For this review, take the finished solid that the model builds, in its own axes (mm). A direction names the side the tool comes from. Coordinates: 2 decimals unless noted, no trailing zeros. Order: outer loops, then holes, each group sorted by start corner. A loop starts at its lowest first (then second) coordinate and runs counter-clockwise, first axis right, second up. Notation, with made-up numbers: (79.5, 36.25) -> (109.5, 36.25) arc R11 cw to (109.5, 44.25) -> close; hole circle Ø11 at (18.5, 41). An arc over 180 degrees is marked (long way). Return JSON: item names as keys, results as strings. Group by question number.
Item 1: Take a section at B-B (x = -55). Write out the cut boundary in (y, z).
Item 2: Take a section at C-C (z = -149). Write out the cut boundary in (x, y), then the cut area to 3 significant figures.
Item 3: Take a section at D-D (z = -42). Write out the cut boundary in (x, y), then the cut area to 3 significant figures.
Item 4: Insertion check: pin 1 (5 mm diameter, centred on x = 42.5, z = -57.5, fed in from +Y); pin 2 (10 mm diameter, centred on x = -15.5, y = -2, fed in from -Z); pin 3 (11 mm diameter, centred on y = 0, z = -42, fed in from -X); pin 4 (12 mm diameter, centred on y = 2, z = -137.5, fed in from +X). Each pin has a flat end and moves straight along its axis. Give the tip position at first contact, or say it passes through.
Item 5: Take a section at A-A (z = -126). Write out the cut boundary in (x, y).
Item 6: Machinability: for faces 4 (the cylindrical face through (39.96, -1.76, -161.75)), 5 (the cylindrical face through (-94, 0, -120)), 6 (the flat face through (-28, 28, -12)), which of the approach directions +Z, -Z, +X, -X, +Y, -Y give a long, thin tool a straight path to every point of the face, cutting with its end or side? Answer none if there is none.
Item 7: For line 1 along Y through (x, z) = (0, -169.5); line 2 along Z through (x, y) = (-28, -46.5); line 3 along Y through (x, z) = (11.5, -62), list the stretches that pass through material, from the lowest coordinate up.
Item 8: Draft analysis for pull direction Y (two halves, no side actions). For faces 1 (the cylindrical face through (-60, 0, -6)), 2 (the flat face through (32, 42, -166)), 3 (the cylindrical face through (-62.952, -19.825, -6.084)), state which applies: +Y half, -Y half, draft (parallel to the pull), parting line (faces both ways), or undercut.
```python
from build123d import *
from build123d.topology import SkipClean

# Parameters (mm, degrees)
SKETCH4_R          = 6
CUT_EXTRUDE1_DEPTH = 12
SKETCH5_R          = 6
CUT_EXTRUDE2_DEPTH = 14
SKETCH14_R         = 6
CUT_EXTRUDE3_DEPTH = 12


with BuildPart() as part:
    # Sketch1 → Revolve1 (revolve)
    with BuildSketch(Plane(origin=(0, 0, 0), x_dir=(1, 0, 0), z_dir=(0, 1, 0)), mode=Mode.PRIVATE) as revolve1_sk:
        Polygon((40, 180), (40, 144), (27, 36), (20, 36), (20, 0), (66, 0), (66, 12), (36, 12), (36, 36), (50, 144), (52, 144), (52, 166), (72, 166), (72, 180), align=None)
    revolve(revolve1_sk.sketch.rotate(Axis((0, 0, -182.979971196), (0, 0, 1)), 180), axis=Axis((0, 0, -182.979971196), (0, 0, 1)))

    # Sketch4 → Cut-Extrude1 (cut)
    with BuildSketch(Plane.XY):
        with Locations((54, 0)):
            Circle(SKETCH4_R)
        with Locations((0, -54)):
            Circle(SKETCH4_R)
        with Locations((-54, 0)):
            Circle(SKETCH4_R)
        with Locations((0, 54)):
            Circle(SKETCH4_R)
    extrude(amount=-CUT_EXTRUDE1_DEPTH, mode=Mode.SUBTRACT)

    # Sketch5 → Cut-Extrude2 (cut)
    with BuildSketch(Plane(origin=(0, 0, -180), x_dir=(-1, 0, 0), z_dir=(0, 0, -1))):
        with Locations((58, 0)):
            Circle(SKETCH5_R)
        with Locations((0, -58)):
            Circle(SKETCH5_R)
        with Locations((-58, 0)):
            Circle(SKETCH5_R)
        with Locations((0, 58)):
            Circle(SKETCH5_R)
    extrude(amount=-CUT_EXTRUDE2_DEPTH, mode=Mode.SUBTRACT)

    # Sketch11 → Revolve2 (revolve)
    with BuildSketch(Plane(origin=(0, 0, 0), x_dir=(1, 0, 0), z_dir=(0, 1, 0)), mode=Mode.PRIVATE) as revolve2_sk:
        Polygon((0, 54.187764991), (-100, 64), (-100, 28), (-88, 28), (-88, 52.774507139), (0, 44.139740331), align=None)
    revolve(revolve2_sk.sketch.rotate(Axis((-156.93032519, 0, -84), (1, 0, 0)), 142.376659073), axis=Axis((-156.93032519, 0, -84), (1, 0, 0)))

    # Sketch12 → Cut-Revolve1 (revolve, cut)
    with BuildSketch(Plane(origin=(0, 0, 0), x_dir=(1, 0, 0), z_dir=(0, 1, 0)), mode=Mode.PRIVATE) as cut_revolve1_sk:
        Polygon((0, 180), (40, 180), (40, 144), (27, 36), (0, 36), align=None)
    revolve(cut_revolve1_sk.sketch.rotate(Axis((0, 0, -182.979971196), (0, 0, 1)), 180), axis=Axis((0, 0, -182.979971196), (0, 0, 1)), mode=Mode.SUBTRACT)

    # Sketch13 → Cut-Revolve2 (revolve, cut)
    with SkipClean():  # the faces are left unmerged after this step: merging them gives an invalid solid
        with BuildSketch(Plane(origin=(0, 0, 0), x_dir=(1, 0, 0), z_dir=(0, 1, 0))):
            Polygon((-100, 64), (0, 54.187764991), (0, 84), (-100, 84), align=None)
        revolve(axis=Axis((-156.93032519, 0, -84), (1, 0, 0)), mode=Mode.SUBTRACT)

    # Sketch14 → Cut-Extrude3 (cut)
    with SkipClean():  # the faces are left unmerged after this step: merging them gives an invalid solid
        with BuildSketch(Plane.ZY.offset(100)):
            with Locations((-42, 0)):
                Circle(SKETCH14_R)
            with Locations(Location((-126, 0, 0), (0, 0, 180))):
                Circle(SKETCH14_R)
            with Locations((-84, 42)):
                Circle(SKETCH14_R)
            with Locations(Location((-84, -42, 0), (0, 0, 180))):
                Circle(SKETCH14_R)
        extrude(amount=-CUT_EXTRUDE3_DEPTH, mode=Mode.SUBTRACT)


solid = part.part
```
Findings below:
{
 "1": {"outline": "(-46.47, -180) -> (-5.2, -180) -> (-5.2, -166) -> (-46.47, -166) -> close; (-36.48, -12) -> (-5.92, -12) -> (-5.92, 0) -> (-36.48, 0) -> close; circle Ø68.93 at (0, -84); (5.2, -180) -> (46.47, -180) -> (46.47, -166) -> (5.2, -166) -> close; (5.92, -12) -> (36.48, -12) -> (36.48, 0) -> (5.92, 0) -> close; hole circle Ø48.83 at (0, -84)"},
 "2": {"outline": "circle Ø104 at (0, 0); hole circle Ø80 at (0, 0)", "area": "3,470 mm2"},
 "3": {"outline": "(-100, -37.04) -> (-88, -37.04) -> (-88, -6) -> (-100, -6) -> close; (-100, 6) -> (-88, 6) -> (-88, 37.04) -> (-100, 37.04) -> close; circle Ø73.56 at (0, 0); hole circle Ø55.44 at (0, 0)", "area": "2,580 mm2"},
 "4": {"pin 1": "passes through", "pin 2": "stops at z = -36", "pin 3": "stops at x = -37.49", "pin 4": "stops at x = 49.91"},
 "5": {"outline": "(-100, -37.04) -> (-88, -37.04) -> (-88, -6) -> (-100, -6) -> close; (-100, 6) -> (-88, 6) -> (-88, 37.04) -> (-100, 37.04) -> close; circle Ø95.33 at (0, 0); hole circle Ø75.67 at (0, 0)"},
 "6": {"face 4": "-Z", "face 5": "-X", "face 6": "none"},
 "7": {"line 1": "y = -72 to -64, -52 to -40, 40 to 52, 64 to 72", "line 2": "z = -180 to -166, -12 to 0", "line 3": "y = -37.65 to -27.85, 27.85 to 37.65"},
 "8": {"face 1": "undercut", "face 2": "draft", "face 3": "parting line"}
}
